```python
from build123d import *

# Parameters (mm, degrees)
SKETCH1_R                                           = 44.45
SKETCH1_R_2                                         = 3.96875
SKETCH1_R_3                                         = 20.6375
BOSS_EXTRUDE1_DEPTH                                 = 25.4
SKETCH2_R                                           = 20.6375
SKETCH2_R_2                                         = 14.2875
BOSS_EXTRUDE2_DEPTH                                 = 14.2875
SKETCH3_R                                           = 20.6375
SKETCH3_R_2                                         = 14.2875
BOSS_EXTRUDE3_DEPTH                                 = 14.2875
CHAMFER1_SIZE                                       = 1.016
CUT_EXTRUDE1_DEPTH                                  = 50.8
CIRPATTERN1_COUNT                                   = 4
CSK_FOR_5_16_FLAT_HEAD_MACHINE_SCREW_10_D           = 8.72998
CSK_FOR_5_16_FLAT_HEAD_MACHINE_SCREW_10_DEPTH       = 50.8
CSK_FOR_5_16_FLAT_HEAD_MACHINE_SCREW_10_CSINK_D     = 16.129
CSK_FOR_5_16_FLAT_HEAD_MACHINE_SCREW_10_CSINK_ANGLE = 100


with BuildPart() as part:
    # Sketch1 → Boss-Extrude1 (new body, symmetric)
    with BuildSketch(Plane.XY):
        Circle(SKETCH1_R)
        with Locations((-25.4, 25.4)):
            Circle(SKETCH1_R_2, mode=Mode.SUBTRACT)
        with Locations((25.4, 25.4)):
            Circle(SKETCH1_R_2, mode=Mode.SUBTRACT)
        with Locations((25.4, -25.4)):
            Circle(SKETCH1_R_2, mode=Mode.SUBTRACT)
        with Locations((-25.4, -25.4)):
            Circle(SKETCH1_R_2, mode=Mode.SUBTRACT)
        Circle(SKETCH1_R_3, mode=Mode.SUBTRACT)
    extrude(amount=BOSS_EXTRUDE1_DEPTH, both=True)

    # Sketch2 → Boss-Extrude2 (add)
    with BuildSketch(Plane.XY):
        Circle(SKETCH2_R)
        Circle(SKETCH2_R_2, mode=Mode.SUBTRACT)
    extrude(amount=BOSS_EXTRUDE2_DEPTH)

    # Sketch3 → Boss-Extrude3 (add)
    with BuildSketch(Plane(origin=(0, 0, 0), x_dir=(-1, 0, 0), z_dir=(0, 0, -1))):
        with Locations(Location((0, 0, 0), (0, 0, 180))):  # turned: the seam where the file's is
            Circle(SKETCH3_R)
        with Locations(Location((0, 0, 0), (0, 0, 180))):  # turned: the seam where the file's is
            Circle(SKETCH3_R_2, mode=Mode.SUBTRACT)
    extrude(amount=BOSS_EXTRUDE3_DEPTH)

    # Chamfer1
    chamfer1_edges = [part.edges().sort_by_distance(p)[0] for p in [
        (-20.6375, 0, -25.4),
        (-20.6375, 0, 25.4),
    ]]
    chamfer(chamfer1_edges, length=CHAMFER1_SIZE)

    # Sketch4 → Cut-Extrude1 (cut)
    with BuildSketch(Plane(origin=(0, 0, -25.4), x_dir=(-1, 0, 0), z_dir=(0, 0, -1))):
        with BuildLine():
            ThreePointArc((-5.392689271, 31.430896424), (-18.411792847, 36.823585695), (-31.430896424, 31.430896424))
            ThreePointArc((-31.430896424, 31.430896424), (0, 44.45), (31.430896424, 31.430896424))
            ThreePointArc((31.430896424, 31.430896424), (18.411792847, 36.823585695), (5.392689271, 31.430896424))
            ThreePointArc((5.392689271, 31.430896424), (0, 29.19717139), (-5.392689271, 31.430896424))
        make_face()
    cut_extrude1 = extrude(amount=-CUT_EXTRUDE1_DEPTH, mode=Mode.SUBTRACT)

    # CirPattern1: Cut-Extrude1 ×4 about axis
    cirpattern1_axis = Axis((0, 0, 0), (0, 0, 1))
    for i in range(1, CIRPATTERN1_COUNT):
        add(cut_extrude1.rotate(cirpattern1_axis, i * 360 / CIRPATTERN1_COUNT), mode=Mode.SUBTRACT)

    # CSK for 5/16 Flat Head Machine Screw (100)1
    with Locations(Plane(origin=(0, 0, -25.4), x_dir=(-1, 0, 0), z_dir=(0, 0, -1))):
        with Locations((25.4, 25.4), (-25.4, 25.4), (-25.4, -25.4), (25.4, -25.4)):
            CounterSinkHole(CSK_FOR_5_16_FLAT_HEAD_MACHINE_SCREW_10_D / 2, CSK_FOR_5_16_FLAT_HEAD_MACHINE_SCREW_10_CSINK_D / 2, depth=CSK_FOR_5_16_FLAT_HEAD_MACHINE_SCREW_10_DEPTH, counter_sink_angle=CSK_FOR_5_16_FLAT_HEAD_MACHINE_SCREW_10_CSINK_ANGLE)


solid = part.part
```
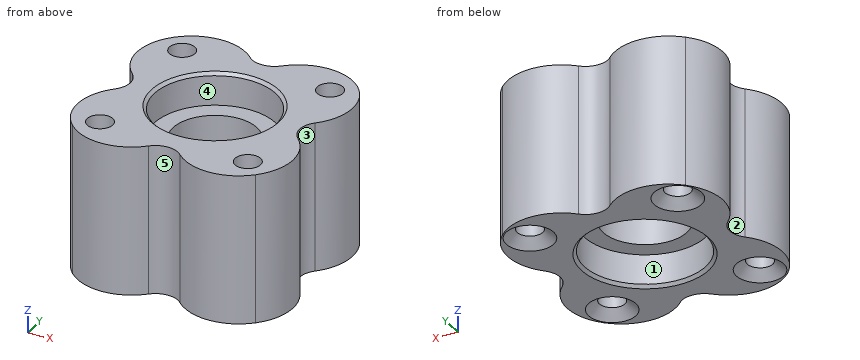
Geometry check sheet. Reference: the model listing, model coordinates, mm. Face numbers are marked on the shaded views. A direction names the side the tool comes from. Give positions to 0.01 mm unless a question says otherwise; leave off trailing zeros. Order: outer loops, then holes, each group sorted by start corner. A loop starts at its lowest first (then second) coordinate and runs counter-clockwise, first axis right, second up. Notation, with made-up numbers: (30.25, -30) - (78.25, -30) arc R30 cw to (78.25, -8) - close; hole circle Ø5 at (58.5, 82.5). An arc over 180 degrees is marked (long way). Answer in a Markdown table with one row per item. Add a question column.
Q1. Tool access check on the marked faces 4 and 5. Record the directions out of +Z, -Z, +X, -X, +Y, -Y that give a thin tool (end or side, any length) a straight path to the whole face; none if there is none.
Q2. Gauge pin test, flat ends, axial feed: pin 1 (1.5 mm diameter, centred on x = 11, z = -16.5, fed in from +Y); pin 2 (5 mm diameter, centred on y = -12, z = 10.5, fed in from -X); pin 3 (10 mm diameter, centred on x = -24, z = 11, fed in from -Y); pin 4 (8 mm diameter, centred on x = -25.4, y = 25.4, fed in from +Z). Record the tip position at first contact, or that the pin passes through.
Q3. Cross-section at B-B, the plane y = 0. Enter the section's corners in (x, z), then the cut area to 3 significant figures.
Q4. Cross-section at C-C, the plane x = 25.4. Enter the section's corners in (y, z).
Q5. Mould release check, pull along X, two halves, no side actions. Record for the marked faces 1, 2 and 3: pulls with the +X half, pulls with the -X half, needs draft (parallel to the pull), parting line crosses it, or undercut.
Q6. Material ranges on probe 1 along X at (y, z) = (0, -6); probe 2 along X at (y, z) = (-25.4, -5.5) (3 decimals); probe 3 along X at (y, z) = (-24, 5), recorded low to high. Write a range as from..to.
Check values:
| question | item | result |
|---|---|---|
| 1 | face 4 | +Z |
| 1 | face 5 | +Z, -Z, -Y |
| 2 | pin 1 | stops at y = 35.58 |
| 2 | pin 2 | stops at x = -36.4 |
| 2 | pin 3 | stops at y = -36.81 |
| 2 | pin 4 | passes through |
| 3 | outline | (-29.2, -25.4) - (-21.65, -25.4) - (-20.64, -24.38) - (-20.64, -14.29) - (-14.29, -14.29) - (-14.29, 14.29) - (-20.64, 14.29) - (-20.64, 24.38) - (-21.65, 25.4) - (-29.2, 25.4) - close; (14.29, -14.29) - (20.64, -14.29) - (20.64, -24.38) - (21.65, -25.4) - (29.2, -25.4) - (29.2, 25.4) - (21.65, 25.4) - (20.64, 24.38) - (20.64, 14.29) - (14.29, 14.29) - close |
| 3 | area | 1,230 mm^2 |
| 4 | outline | (-35.45, -25.4) - (-33.46, -25.4) - (-29.76, -22.3) - (-29.76, 25.4) - (-35.45, 25.4) - close; (-21.04, -22.3) - (-17.34, -25.4) - (17.34, -25.4) - (21.04, -22.3) - (21.04, 25.4) - (-21.04, 25.4) - close; (29.76, -22.3) - (33.46, -25.4) - (35.45, -25.4) - (35.45, 25.4) - (29.76, 25.4) - close |
| 5 | face 1 | undercut |
| 5 | face 2 | pulls with the -X half |
| 5 | face 3 | pulls with the +X half |
| 6 | probe 1 | x = -29.2..-14.29, 14.29..29.2 |
| 6 | probe 2 | x = -35.446..-29.765, -21.035..21.035, 29.765..35.446 |
| 6 | probe 3 | x = -35.96..-29.53, -21.27..21.27, 29.53..35.96 |
